Check sheet for the modelled part. Datum: model origin and axes. Units: mm. A direction names the side the tool comes from. Coordinates: 2 decimals unless noted, no trailing zeros. Loops run counter-clockwise (first coordinate to the right, second up) from the corner with the lowest first, then second, coordinate; pieces in that order, holes last. Notation, with made-up numbers: M 59,52 L 118,52 A37 cw 118,90 Z; hole C -19,-18.75 d4. An arc over 180 degrees is marked long. Write each question's results on one line, items separated by ' | '. Start each with the question number.
from build123d import *

# Parameters (mm, degrees)
SKETCH2_W           = 210
SKETCH2_H           = 180
BOSS_EXTRUDE1_DEPTH = 5
SKETCH3_W           = 90
SKETCH3_H           = 5
BOSS_EXTRUDE2_DEPTH = 20
SKETCH4_W           = 90
SKETCH4_H           = 5
BOSS_EXTRUDE3_DEPTH = 20
SKETCH5_R           = 1.65
SKETCH5_R_2         = 2.2
CUT_EXTRUDE1_DEPTH  = 153.151240547


with BuildPart() as part:
    # Sketch2 → Boss-Extrude1 (new body)
    with BuildSketch(Plane.XY):
        Rectangle(SKETCH2_W, SKETCH2_H)
    extrude(amount=BOSS_EXTRUDE1_DEPTH)

    # Sketch3 → Boss-Extrude2 (add)
    with BuildSketch(Plane(origin=(0, -90, 0), x_dir=(-1, 0, 0), z_dir=(0, -1, 0))):
        with Locations((0, -2.5)):
            Rectangle(SKETCH3_W, SKETCH3_H)
    extrude(amount=BOSS_EXTRUDE2_DEPTH)

    # Sketch4 → Boss-Extrude3 (add)
    with BuildSketch(Plane(origin=(0, 90, 0), x_dir=(1, 0, 0), z_dir=(0, 1, 0))):
        with Locations((0, -2.5)):
            Rectangle(SKETCH4_W, SKETCH4_H)
    extrude(amount=BOSS_EXTRUDE3_DEPTH)

    # Sketch5 → Cut-Extrude1 (cut, through all)
    with BuildSketch(Plane.XY.offset(5)):
        with Locations((89.5, 83.5)):
            Circle(SKETCH5_R)
        with Locations((89.5, 77.5)):
            Circle(SKETCH5_R)
        with Locations((89.5, 71.5)):
            Circle(SKETCH5_R)
        with Locations((60.5, 83.5)):
            Circle(SKETCH5_R)
        with Locations((60.5, 77.5)):
            Circle(SKETCH5_R)
        with Locations((60.5, 71.5)):
            Circle(SKETCH5_R)
        with Locations(Location((-60.5, 71.5, 0), (0, 0, 180))):
            Circle(SKETCH5_R)
        with Locations(Location((-60.5, 77.5, 0), (0, 0, 180))):
            Circle(SKETCH5_R)
        with Locations(Location((-60.5, 83.5, 0), (0, 0, 180))):
            Circle(SKETCH5_R)
        with Locations(Location((-89.5, 71.5, 0), (0, 0, 180))):
            Circle(SKETCH5_R)
        with Locations(Location((-89.5, 77.5, 0), (0, 0, 180))):
            Circle(SKETCH5_R)
        with Locations(Location((-89.5, 83.5, 0), (0, 0, 180))):
            Circle(SKETCH5_R)
        with Locations((-89.5, -83.5)):
            Circle(SKETCH5_R)
        with Locations((-89.5, -77.5)):
            Circle(SKETCH5_R)
        with Locations((-89.5, -71.5)):
            Circle(SKETCH5_R)
        with Locations((-60.5, -83.5)):
            Circle(SKETCH5_R)
        with Locations((-60.5, -77.5)):
            Circle(SKETCH5_R)
        with Locations((-60.5, -71.5)):
            Circle(SKETCH5_R)
        with Locations(Location((60.5, -71.5, 0), (0, 0, 180))):
            Circle(SKETCH5_R)
        with Locations(Location((60.5, -77.5, 0), (0, 0, 180))):
            Circle(SKETCH5_R)
        with Locations(Location((60.5, -83.5, 0), (0, 0, 180))):
            Circle(SKETCH5_R)
        with Locations(Location((89.5, -71.5, 0), (0, 0, 180))):
            Circle(SKETCH5_R)
        with Locations(Location((89.5, -77.5, 0), (0, 0, 180))):
            Circle(SKETCH5_R)
        with Locations(Location((89.5, -83.5, 0), (0, 0, 180))):
            Circle(SKETCH5_R)
        with Locations((45, 25)):
            Circle(SKETCH5_R_2)
        with Locations((45, -25)):
            Circle(SKETCH5_R_2)
        with Locations((-75, 25)):
            Circle(SKETCH5_R_2)
        with Locations((-75, -25)):
            Circle(SKETCH5_R_2)
    extrude(amount=-CUT_EXTRUDE1_DEPTH, mode=Mode.SUBTRACT)


solid = part.part
1) Thickness scan on probe 1 along X at (y, z) = (77.5, 1.1); probe 2 along X at (y, z) = (27, 0.6); probe 3 along Y at (x, z) = (-45.5, 0.7). Record the ranges inside material, lowest first.
2) Set-up check for faces 1 (the flat face through (-75, 90, 2)), 2 (the flat face through (-45, -100, 3)), 3 (the flat face through (-1, 2, 5)), 4 (the flat face through (45, 100, 3)), 5 (the flat face through (45, -100, 3)): record each of +Z, -Z, +X, -X, +Y, -Y from which the full face is reachable in a straight line by a thin tool's end or side.
3) Section check B-B (x = -69.5). Enter the section's corners in (y, z).
4) Gauge pin test, flat end, axial feed: P1, Ø2.5, axis at y = -96, z = 1.5, coming from the -X side. Record the tip position at first contact, or that the pin passes through.
5) Section check A-A (z = 4). Give the number of separate pieces and of enclosed holes in the cut face, then the cut area to 3 significant figures.
Return value:
1) probe 1: x = -105 to -91.15, -87.85 to -62.15, -58.85 to 58.85, 62.15 to 87.85, 91.15 to 105 | probe 2: x = -105 to -75.92, -74.08 to 44.08, 45.92 to 105 | probe 3: y = -90 to 90
2) face 1: +Z, -Z, -X, +Y | face 2: +Z, -Z, -X, -Y | face 3: +Z, +X, -X, +Y, -Y | face 4: +Z, -Z, +X, +Y | face 5: +Z, -Z, +X, -Y
3) outline: M -90,0 L 90,0 L 90,5 L -90,5 Z
4) P1: stops at x = -45
5) separate pieces: 1 | enclosed holes: 28 | area: 41,100 mm2
